Can you work these out from the model? Positions are in its coordinate system, mm. A direction names the side the tool comes from. Give positions to 0.01 mm unless a question says otherwise; leave off trailing zeros. Order: outer loops, then holes, each group sorted by start corner. A loop starts at its lowest first (then second) coordinate and runs counter-clockwise, first axis right, second up. Notation, with made-up numbers: (-17, 47.25) - (-11, 47.25) arc R10 cw to (-11, 56.25) - close; hole circle Ø6 at (-17.5, -15.75). An arc over 180 degrees is marked (long way). Write each question's results on one line, items separated by ' | '. Start each with the question number.
from build123d import *

# Parameters (mm, degrees)
SKETCH1_R           = 9.525
BOSS_EXTRUDE1_DEPTH = 114.3
SKETCH2_R           = 5.55625
CUT_EXTRUDE1_DEPTH  = 101.6
SKETCH3_R           = 3.175
CUT_EXTRUDE2_DEPTH  = 114.3
CUT_EXTRUDE8_DEPTH  = 7.62
CUT_REVOLVE1_ANGLE  = 75
SKETCH8_R           = 9.525
SKETCH8_R_2         = 9.4742
CUT_EXTRUDE10_DEPTH = 25.4


with BuildPart() as part:
    # Sketch1 → Boss-Extrude1 (new body)
    with BuildSketch(Plane.XY):
        Circle(SKETCH1_R)
    extrude(amount=BOSS_EXTRUDE1_DEPTH)

    # Sketch2 → Cut-Extrude1 (cut)
    with BuildSketch(Plane(origin=(0, 0, 0), x_dir=(-1, 0, 0), z_dir=(0, 0, -1))):
        Circle(SKETCH2_R)
    extrude(amount=-CUT_EXTRUDE1_DEPTH, mode=Mode.SUBTRACT)

    # Sketch3 → Cut-Extrude2 (cut)
    with BuildSketch(Plane.XY.offset(114.3)):
        Circle(SKETCH3_R)
    extrude(amount=-CUT_EXTRUDE2_DEPTH, mode=Mode.SUBTRACT)

    # Sketch5 → Cut-Extrude8 (cut)
    with BuildSketch(Plane.XY.offset(114.3)):
        with BuildLine():
            ThreePointArc((9.525, 0), (9.49163573, 0.796540129), (9.391776656, 1.5875))
            Line((9.391776656, 1.5875), (6.35, 1.5875))
            Line((6.35, 1.5875), (6.35, -1.5875))
            Line((6.35, -1.5875), (9.391776656, -1.5875))
            ThreePointArc((9.391776656, -1.5875), (9.49163573, -0.796540129), (9.525, 0))
        make_face()
        with BuildLine():
            Line((-6.35, 1.5875), (-9.391776656, 1.5875))
            ThreePointArc((-9.391776656, 1.5875), (-9.525, 0), (-9.391776656, -1.5875))
            Line((-9.391776656, -1.5875), (-6.35, -1.5875))
            Line((-6.35, -1.5875), (-6.35, 1.5875))
        make_face()
    extrude(amount=-CUT_EXTRUDE8_DEPTH, mode=Mode.SUBTRACT)

    # Sketch7 → Cut-Revolve1 (revolve, cut)
    with BuildSketch(Plane(origin=(0, 0, 0), x_dir=(1, 0, 0), z_dir=(0, 1, 0))):
        Polygon((9.391776656, -106.68), (6.35, -106.68), (6.35, -109.855), (9.525, -109.855), (9.525, -106.68), align=None)
        Polygon((-6.35, -109.855), (-9.525, -109.855), (-9.525, -106.68), (-9.391776656, -106.68), (-6.35, -106.68), align=None)
    revolve(axis=Axis((0, 0, 0), (0, 0, 1)), revolution_arc=CUT_REVOLVE1_ANGLE, mode=Mode.SUBTRACT)

    # Sketch8 → Cut-Extrude10 (cut)
    with BuildSketch(Plane.XY.offset(114.3)):
        Circle(SKETCH8_R)
        Circle(SKETCH8_R_2, mode=Mode.SUBTRACT)
    extrude(amount=-CUT_EXTRUDE10_DEPTH, mode=Mode.SUBTRACT)


solid = part.part
Q1. Which directions (+Z, -Z, +X, -X, +Y, -Y) give clear straight access to the entire face, cutting with the end or side of a thin tool? Please do faces 5 (the flat face through (6.35, 0, 111)), 6 (the flat face through (2.04, 7.62, 108.25)), 7 (the flat face through (-6.35, 0, 111)), 8 (the flat face through (-2.04, -7.62, 108.25)).
Q2. If we section it at A-A (x = 0): Please give me the cut outline in (y, z) (3 decimals), plus the area to 3 significant figures.
Q3. If we section it at C-C (y = -4.25): Please give me the cut outline in (x, z) (3 decimals).
Q4. Thinking about a two-plate mould opening in Y: for faces 1 (the cylindrical face through (-0.69, -3.1, 108.04)), 2 (the cylindrical face through (-7.559, -5.796, 43.828)), 3 (the flat face through (-8, 1.588, 111)), 4 (the flat face through (4.1, -4.1, 0)), which applies, released by +Y, released by -Y, zero draft, split by the parting line, or undercut?
Q5. Will these pins go through, and if not, where does the flat tip stop? P1, Ø3.5, axis at y = -1, z = 109.5, coming from the +X side; P2, Ø1.5, axis at y = 6, z = 72.5, coming from the -X side; P3, Ø1, axis at y = 5.5, z = 51, coming from the +X side; P4, Ø5, axis at x = 0, y = 0, coming from the +Z side.
Q6. If I drill on probe 1 along Z at (x, y) = (-7.5, -3.5) (3 decimals); probe 2 along Y at (x, z) = (0, 49) (3 decimals); probe 3 along Y at (x, z) = (0, 111.5) (3 decimals), over which ranges is the centre line in solid material (lowest first)? Write a range as from..to.
Findings below:
1) face 5: +Z, +X | face 6: +X | face 7: +Z, -X | face 8: -X
2) outline: (-9.525, 0) - (-5.556, 0) - (-5.556, 101.6) - (-3.175, 101.6) - (-3.175, 114.3) - (-9.474, 114.3) - (-9.474, 88.9) - (-9.525, 88.9) - close; (3.175, 101.6) - (5.556, 101.6) - (5.556, 0) - (9.525, 0) - (9.525, 88.9) - (9.474, 88.9) - (9.474, 114.3) - (3.175, 114.3) - close | area: 965 mm2
3) outline: (-8.524, 0) - (-3.579, 0) - (-3.579, 101.6) - (3.579, 101.6) - (3.579, 0) - (8.524, 0) - (8.524, 88.9) - (8.467, 88.9) - (8.467, 114.3) - (-8.467, 114.3) - (-8.467, 109.855) - (-4.718, 109.855) - (-4.718, 106.68) - (-8.467, 106.68) - (-8.467, 88.9) - (-8.524, 88.9) - close
4) face 1: undercut | face 2: split by the parting line | face 3: undercut | face 4: zero draft
5) P1: stops at x = 9.34 | P2: stops at x = -7.95 | P3: stops at x = 8.11 | P4: passes through
6) probe 1: z = 0..106.68, 109.855..114.3 | probe 2: y = -9.525..-5.556, 5.556..9.525 | probe 3: y = -9.474..-3.175, 3.175..9.474
